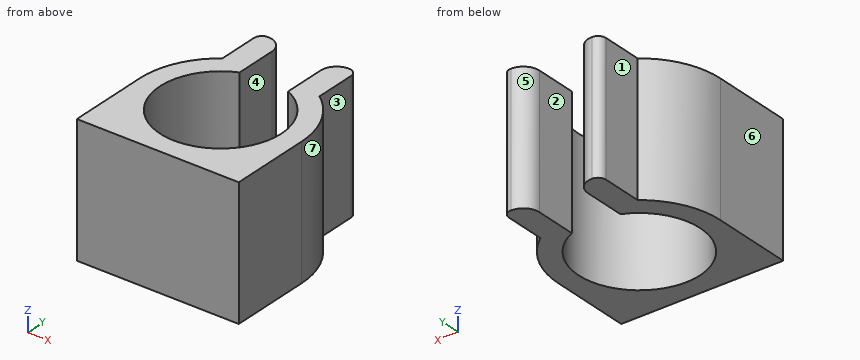
Autodesk Inventor part; units mm, degrees
ref_plane "YZ Plane" through (0, 0, 0) normal (1, 0, 0) x (0, 1, 0)
ref_plane "XZ Plane" through (0, 0, 0) normal (0, 1, 0) x (-1, 0, 0)
ref_plane "XY Plane" through (0, 0, 0) normal (0, 0, 1) x (1, 0, 0)
sketch "Sketch3" plane through (0, 0, 0) normal (0, 0, 1) x (1, 0, 0)
  line L0 (0, 0) -> (-5, 0)
  line L1 (-5, 0) -> (-5, 5)
  line L2 (0, 0) -> (5, 0)
  line L3 (5, 0) -> (5, 5)
  arc A0 (-1.5, 8.4369) -> (1.5, 8.4369) centre (0, 5) ccw
  line L4 (-3, 9) -> (-3, 12)
  line L5 (-3, 12) -> (-1.5, 12)
  line L6 (-1.5, 12) -> (-1.5, 9.7697)
  line L7 (1.5, 9.7697) -> (1.5, 12)
  line L8 (1.5, 12) -> (3, 12)
  line L9 (3, 12) -> (3, 9)
  line L10 (-1.5, 9.7697) -> (-1.5, 8.4369)
  line L11 (1.5, 9.7697) -> (1.5, 8.4369)
  arc A1 (-3, 9) -> (-5, 5) centre (0, 5) ccw
  arc A2 (5, 5) -> (3, 9) centre (0, 5) ccw
  dimension "d9" = 5
  dimension "d10" = 7.5
  dimension "d11" = 3
  dimension "d12" = 7
  dimension "d13" = 1.5
  dimension "d14" = 5
  dimension "d15" = 5
  dimension "d16" = 1.5
extrude "Extrusion1" add sketch "Sketch3" along normal blind 8
fillet "Fillet1" radius 1 2 edges at (-1.5, 12, 4) (1.5, 12, 4)
fillet "Fillet2" radius 0.5 2 edges at (3, 12, 4) (-3, 12, 4)
properties part number "WireClip"
Geometry: final body of the model. Coordinates: model frame, mm. Face numbers are marked on the shaded views. A direction names the side the tool comes from. Coordinates: 2 decimals unless noted, no trailing zeros. Write each loop counter-clockwise with the first axis right and the second up, starting at its lowest first coordinate (ties: lowest second). Pieces come first, ordered by that corner, then holes. Notation, with made-up numbers: M 20,28 L 55,28 A30 ccw 55,54 Z; hole C 33,-34.75 d7. An arc over 180 degrees is marked long. Use CSV: the item, a comma, the result in double quotes. Start each with the question number.
1. Ray query, probe 1 along X at (y, z) = (10, 7.75); probe 2 along X at (y, z) = (5, 3); probe 3 along Y at (x, z) = (0, 6). Return the intervals inside material, ascending.
2. Cut plane D-D on x = 0. Return the cut outline in (y, z).
3. Cut plane A-A on y = 9.25. Return the cut outline in (x, z).
4. Cut plane B-B on x = -1.75. Return the cut outline in (y, z).
5. Mould query, pull axis X, two halves, no side actions, for the marked faces 4, 5, 6 and 7. Classes: pulls with the +X half, pulls with the -X half, needs draft (parallel to the pull), parting line crosses it, or undercut.
6. Reachability of the marked faces 1, 2 and 3 from +Z, -Z, +X, -X, +Y, -Y: full face, straight path, thin tool, end or side. Return the list, or none.
7. First-contact query: P1, Ø3, axis at y = 9.5, z = 5.5, coming from the -X side; P2, Ø4, axis at x = 4, z = 3.5, coming from the +Y side; P3, Ø2, axis at y = 10.5, z = 3, coming from the -X side; P4, Ø0.8, axis at y = 9.5, z = 5, coming from the +X side. Flat tips, straight axial feed; report the tip coordinate or a pass-through.
Entries:
1,probe 1,"-3 to -1.5, 1.5 to 3"
1,probe 2,"-5 to -3.75, 3.75 to 5"
1,probe 3,"0 to 1.25"
2,outline,"M 0,0 L 1.25,0 L 1.25,8 L 0,8 Z"
3,outline,"M -3,0 L -1.5,0 L -1.5,8 L -3,8 Z; M 1.5,0 L 3,0 L 3,8 L 1.5,8 Z"
4,outline,"M 0,0 L 1.68,0 L 1.68,8 L 0,8 Z; M 8.32,0 L 11.66,0 L 11.66,8 L 8.32,8 Z"
5,face 4,"undercut"
5,face 5,"undercut"
5,face 6,"pulls with the -X half"
5,face 7,"pulls with the +X half"
6,face 1,"+Z, -Z, -X, +Y"
6,face 2,"+Z, -Z, +Y"
6,face 3,"+Z, -Z, +X, +Y"
7,P1,"x = -4"
7,P2,"y = 12"
7,P3,"x = -3"
7,P4,"x = 3"
